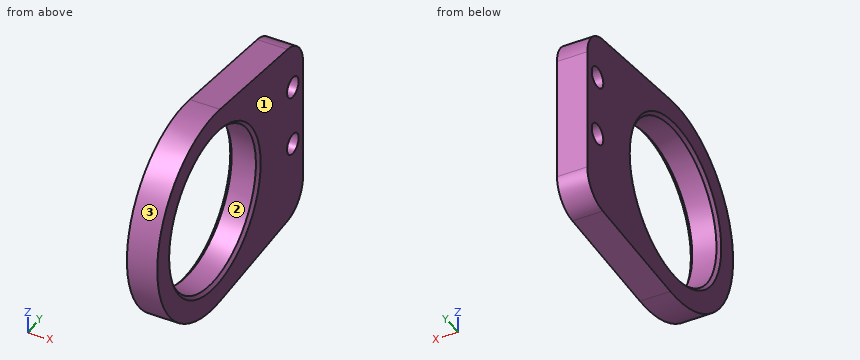
from build123d import *

# Parameters (mm, degrees)
SKETCH_1_R         = 17
SKETCH_1_R_2       = 13
SKETCH_1_W         = 30
SKETCH_1_H         = 3
EXTRUDE_1_DEPTH    = 5
FILLET_1_R         = 5
HOLE_WIZARD_M3_1_D = 3.4
CHAMFER1_SIZE      = 0.5


with BuildPart() as part:
    # 草图1 → 凸台-拉伸1 (new body)
    with BuildSketch(Plane(origin=(0, 0, 0), x_dir=(0, 0, -1), z_dir=(1, 0, 0))):
        Circle(SKETCH_1_R)
        Circle(SKETCH_1_R_2, mode=Mode.SUBTRACT)
        with BuildLine():
            Line((15, 23), (-15, 23))
            Line((-15, 23), (-16.931656145, 1.522832949))
            ThreePointArc((-16.931656145, 1.522832949), (0, 17), (16.931656145, 1.522832949))
            Line((16.931656145, 1.522832949), (15, 23))
        make_face()
        with Locations((0, 24.5)):
            Rectangle(SKETCH_1_W, SKETCH_1_H)
    extrude(amount=EXTRUDE_1_DEPTH)

    # 圆角1
    fillet_1_edges = [part.edges().sort_by_distance(p)[0] for p in [
        (2.5, 26, 15),
        (2.5, 26, -15),
    ]]
    fillet(fillet_1_edges, radius=FILLET_1_R)

    # M3 间隙孔1 (through all)
    with Locations(Plane.ZY):
        with Locations((-2.5, 23), (7.5, 23)):
            Hole(HOLE_WIZARD_M3_1_D / 2)

    # Chamfer1
    chamfer1_edges = [part.edges().sort_by_distance(p)[0] for p in [
        (0, 0, 13),
        (5, 0, 13),
    ]]
    chamfer(chamfer1_edges, length=CHAMFER1_SIZE)


solid = part.part
Verification items for the finished model (mm, model axes). Face numbers are marked on the shaded views. Coordinates: 2 decimals unless noted, no trailing zeros. Order: outer loops, then holes, each group sorted by start corner. A loop starts at its lowest first (then second) coordinate and runs counter-clockwise, first axis right, second up. Notation, with made-up numbers: M 2,65.25 L 38,65.25 A24 ccw 38,96.25 Z; hole C 28.5,48 d9. An arc over 180 degrees is marked long. One line per item, written item: value. Start each with the question number.
Item 1: Sectioned sample at B-B (z = 0). Enter the section's corners in (x, y).
Item 2: Mould release check, pull along Z, two halves, no side actions. Record for the marked faces 1, 2 and 3: released by +Z, released by -Z, zero draft, split by the parting line, or undercut.
Item 3: Sectioned sample at A-A (y = 0). Enter the section's corners in (x, z), then the cut area to 3 significant figures.
Item 4: Scan lines: probe 1 along Y at (x, z) = (2.95, 6); probe 2 along Y at (x, z) = (3.4, 0); probe 3 along Y at (x, z) = (1.8, 8). Record each from-to range of solid material in increasing order.
Item 5: Gauge pin test, flat ends, axial feed: pin 1 (1 mm diameter, centred on x = 2.5, z = 13.5, fed in from -Y); pin 2 (1.5 mm diameter, centred on x = 2, y = -1, fed in from +Z); pin 3 (1 mm diameter, centred on x = 1, y = -4, fed in from -Z). Record the tip position at first contact, or that the pin passes through.
Item 6: Sectioned sample at C-C (x = 2.65). Count the separate pieces of the cut face and the enclosed holes in it, then the cut area to 3 significant figures.
Conclusion:
1. outline: M 0,-17 L 5,-17 L 5,-13.5 L 4.5,-13 L 0.5,-13 L 0,-13.5 Z; M 0,13.5 L 0.5,13 L 4.5,13 L 5,13.5 L 5,26 L 0,26 Z
2. face 1: zero draft
2. face 2: undercut
2. face 3: split by the parting line
3. outline: M 0,-17 L 5,-17 L 5,-13.5 L 4.5,-13 L 0.5,-13 L 0,-13.5 Z; M 0,13.5 L 0.5,13 L 4.5,13 L 5,13.5 L 5,17 L 0,17 Z
3. area: 39.5 mm^2
4. probe 1: y = -15.91 to -11.53, 11.53 to 22.2, 23.8 to 26
4. probe 2: y = -17 to -13, 13 to 26
4. probe 3: y = -15 to -10.25, 10.25 to 21.38, 24.62 to 26
5. pin 1: stops at y = -10.95
5. pin 2: stops at z = 17
5. pin 3: stops at z = -16.64
6. separate pieces: 1
6. enclosed holes: 3
6. area: 723 mm^2
